Source: three-view drawing plus pictorial views. Frame: mm from the lowest corner of the part. A direction names the side the tool comes from. Give positions to 0.01 mm unless a question says otherwise; leave off trailing zeros. One line per question, with ' | ' between items. Start each with the question number.
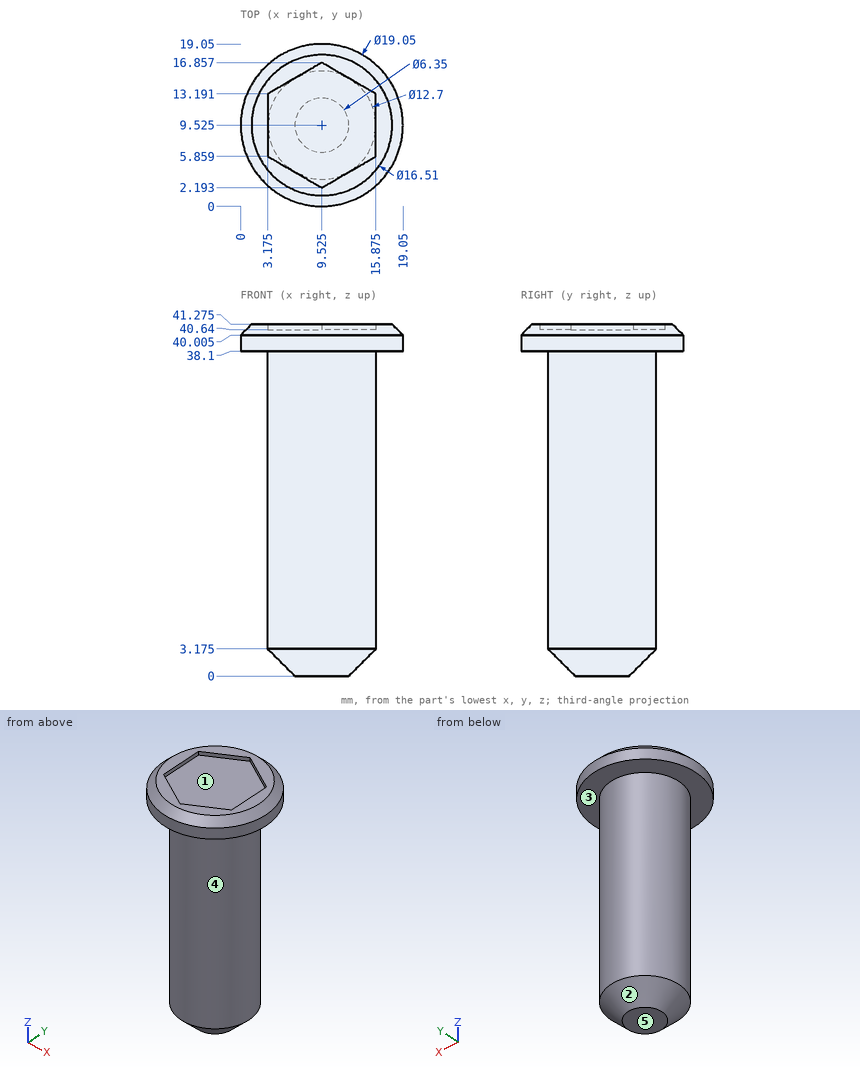
Item 1: Reachability of the marked faces 4 and 5 from +Z, -Z, +X, -X, +Y, -Y: full face, straight path, thin tool, end or side. Return the list, or none.
Item 2: Line query: line 1 (Z direction, x = 11.5, y = 12); line 2 (X direction, y = 14.5, z = 33); line 3 (Y direction, x = 13.25, z = 14). Output: solid intervals per line, ascending.
Item 3: Pin query (flat end, axial travel): pin 1 Ø4 at (x, y) = (8.5, 13.5) entering from +Z; pin 2 Ø1.5 at (y, z) = (12.5, 31) entering from +X; pin 3 Ø1.5 at (y, z) = (12, 31) entering from +X. Return the tip coordinate at first contact, or that it passes through.
Item 4: Mould query, pull axis X, two halves, no side actions, for the marked faces 1, 2 and 3. Classes: pulls with the +X half, pulls with the -X half, needs draft (parallel to the pull), parting line crosses it, or undercut.
Results are:
1) face 4: -Z | face 5: -Z, +X, -X, +Y, -Y
2) line 1: z = 0 to 40.64 | line 2: x = 5.58 to 13.47 | line 3: y = 4.38 to 14.67
3) pin 1: stops at z = 40.64 | pin 2: stops at x = 15.47 | pin 3: stops at x = 15.64
4) face 1: undercut | face 2: parting line crosses it | face 3: needs draft
